Source: CAD feature listing. Evaluate the final solid. Frame: model axes, mm. Face numbers are marked on the shaded views. A direction names the side the tool comes from. Round coordinates to 2 decimals unless told otherwise and drop trailing zeros. Loops run counter-clockwise (first coordinate to the right, second up) from the corner with the lowest first, then second, coordinate; pieces in that order, holes last. Notation, with made-up numbers: (50.5, 89) -> (56.5, 89) arc R18 cw to (56.5, 98) -> close; hole circle Ø2 at (-24, -14.75). An arc over 180 degrees is marked (long way). Write item = value, one per line.
from build123d import *

# Parameters (mm, degrees)
SKETCH1_W               = 54
SKETCH1_H               = 60
BOSS_EXTRUDE1_DEPTH     = 5
BOSS_EXTRUDE2_DEPTH     = 54
SKETCH6_W               = 9.25
SKETCH6_H               = 32
CUT_EXTRUDE1_DEPTH      = 99.244592727
SKETCH8_W               = 9.25
SKETCH8_H               = 42
CUT_EXTRUDE3_DEPTH      = 99.244592727
M4_CLEARANCE_HOLE2_D    = 4.3
CUT_EXTRUDE4_DEPTH      = 94.480278669
SKETCH12_W              = 21.2
SKETCH12_H              = 46
CUT_EXTRUDE5_DEPTH      = 99.244592727
CHAMFER1_SIZE           = 2
CHAMFER2_SIZE           = 5
CHAMFER2_SIZE_2         = 5.352523158
SKETCH13_W              = 21.2
SKETCH13_H              = 5
CUT_EXTRUDE6_DEPTH      = 99.244592727
CHAMFER3_SIZE           = 5
BOSS_EXTRUDE3_DEPTH     = 19
CUT_EXTRUDE7_DEPTH      = 94.480278669
CUT_EXTRUDE7_DEPTH_BACK = 94.480278669
CHAMFER4_SIZE           = 0.4
CHAMFER5_SIZE           = 0.4


with BuildPart() as part:
    # Sketch1 → Boss-Extrude1 (new body)
    with BuildSketch(Plane.XY):
        with Locations((27, 30)):
            Rectangle(SKETCH1_W, SKETCH1_H)
    extrude(amount=BOSS_EXTRUDE1_DEPTH)

    # Sketch5 → Boss-Extrude2 (add)
    with BuildSketch(Plane.ZY):
        Polygon((56, 60), (5, 60), (5, 0), (56, 51), align=None)
    extrude(amount=-BOSS_EXTRUDE2_DEPTH)

    # Sketch6 → Cut-Extrude1 (cut, through all)
    with BuildSketch(Plane(origin=(0, 60, 0), x_dir=(1, 0, 0), z_dir=(0, 1, 0))):
        with Locations((4.625, -21)):
            Rectangle(SKETCH6_W, SKETCH6_H)
    cut_extrude1 = extrude(amount=-CUT_EXTRUDE1_DEPTH, mode=Mode.SUBTRACT)

    # Sketch8 → Cut-Extrude3 (cut, through all)
    with BuildSketch(Plane(origin=(0, 0, 0), x_dir=(-1, 0, 0), z_dir=(0, 0, -1))):
        with Locations((-4.625, 30)):
            Rectangle(SKETCH8_W, SKETCH8_H)
    cut_extrude3 = extrude(amount=-CUT_EXTRUDE3_DEPTH, mode=Mode.SUBTRACT)

    # Mirror1: Cut-Extrude1, Cut-Extrude3 across plane
    add(cut_extrude1.mirror(Plane(origin=(27, 0, 0), x_dir=(0, 0, 1), z_dir=(1, 0, 0))), mode=Mode.SUBTRACT)
    add(cut_extrude3.mirror(Plane(origin=(27, 0, 0), x_dir=(0, 0, 1), z_dir=(1, 0, 0))), mode=Mode.SUBTRACT)

    # M4 Clearance Hole2 (through all)
    with Locations(Plane(origin=(0, 0, 0), x_dir=(-1, 0, 0), z_dir=(0, 0, -1))):
        with Locations((-4.5, 55.5), (-49.5, 55.5), (-49.5, 4.5), (-4.5, 4.5)):
            Hole(M4_CLEARANCE_HOLE2_D / 2)

    # Sketch11 → Cut-Extrude4 (cut, through all)
    with BuildSketch(Plane.ZY.offset(-9.25)):
        Polygon((0, 9), (37, 51), (0, 51), align=None)
    extrude(amount=-CUT_EXTRUDE4_DEPTH, mode=Mode.SUBTRACT)

    # Sketch12 → Cut-Extrude5 (cut, through all)
    with BuildSketch(Plane(origin=(0, 60, 0), x_dir=(1, 0, 0), z_dir=(0, 1, 0))):
        with Locations((27, -28)):
            Rectangle(SKETCH12_W, SKETCH12_H)
    extrude(amount=-CUT_EXTRUDE5_DEPTH, mode=Mode.SUBTRACT)

    # Chamfer1
    chamfer1_edges = [part.edges().sort_by_distance(p)[0] for p in [
        (0, 60, 2.5),
        (0, 9, 2.5),
        (0, 51, 2.5),
        (0, 51, 46.5),
        (54, 60, 2.5),
        (0, 60, 46.5),
        (54, 60, 46.5),
        (54, 0, 2.5),
        (0, 0, 2.5),
        (54, 51, 46.5),
        (54, 9, 2.5),
        (54, 51, 2.5),
    ]]
    chamfer(chamfer1_edges, length=CHAMFER1_SIZE)

    # Chamfer2
    # the kernel refuses this chamfer: 5.352523158, 5 mm, written as the material it adds along each edge
    with BuildSketch(Plane(origin=(37.6, 51, 37), x_dir=(0, -0.7759635654606418, -0.6307777303278932), z_dir=(1, 0, 0)), Plane(origin=(9.25, 51, 37), x_dir=(0, -0.7759635654606418, -0.6307777303278932), z_dir=(1, 0, 0))) as chamfer2_piece_1:
        Polygon((CHAMFER2_SIZE * 0.999214586642, CHAMFER2_SIZE * 0.039625873385), (CHAMFER2_SIZE_2 * 0.630777730356, CHAMFER2_SIZE_2 * 0.775963565495), (0, 0), align=None)
    extrude(amount=7.15)

    # Sketch13 → Cut-Extrude6 (cut, through all)
    with BuildSketch(Plane(origin=(0, 0, 0), x_dir=(-1, 0, 0), z_dir=(0, 0, -1))):
        with Locations((-27, 48.5)):
            Rectangle(SKETCH13_W, SKETCH13_H)
    extrude(amount=-CUT_EXTRUDE6_DEPTH, mode=Mode.SUBTRACT)

    # Chamfer3
    chamfer3_edges = [part.edges().sort_by_distance(p)[0] for p in [
        (16.4, 55.5, 5),
        (16.4, 7.337837838, 5),
        (37.6, 7.337837838, 5),
        (37.6, 55.5, 5),
        (16.4, 55.5, 51),
        (37.6, 55.5, 51),
    ]]
    chamfer(chamfer3_edges, length=CHAMFER3_SIZE)

    # Sketch14 → Boss-Extrude3 (add)
    with BuildSketch(Plane(origin=(0, 0, 37), x_dir=(-1, 0, 0), z_dir=(0, 0, -1))):
        Polygon((-2, 51), (-9.25, 43.75), (-9.25, 51), align=None)
    boss_extrude3 = extrude(amount=-BOSS_EXTRUDE3_DEPTH)

    # Mirror3: Boss-Extrude3 across plane
    add(boss_extrude3.mirror(Plane(origin=(27, 0, 0), x_dir=(0, 0, 1), z_dir=(1, 0, 0))))

    # Sketch15 → Cut-Extrude7 (cut, two sides: drawn at the far end of the back side and taken through both)
    with BuildSketch(Plane(origin=(9.25, 0, 0), x_dir=(0, 0, -1), z_dir=(1, 0, 0)).offset(-CUT_EXTRUDE7_DEPTH_BACK)):
        Polygon((-48.75, 43.75), (-56, 51), (-56, 43.75), align=None)
    extrude(amount=CUT_EXTRUDE7_DEPTH + CUT_EXTRUDE7_DEPTH_BACK, mode=Mode.SUBTRACT)

    # Chamfer4
    chamfer4_edges = [part.edges().sort_by_distance(p)[0] for p in [
        (47.35, 55.5, 37),
        (47.35, 55.5, 56),
        (2.35, 55.5, 56),
        (2.35, 55.5, 37),
    ]]
    chamfer(chamfer4_edges, length=CHAMFER4_SIZE)

    # Chamfer5
    chamfer5_edges = [part.edges().sort_by_distance(p)[0] for p in [
        (2.35, 4.5, 5),
        (2.35, 4.5, 0),
        (47.35, 4.5, 5),
        (47.35, 4.5, 0),
        (47.35, 55.5, 5),
        (47.35, 55.5, 0),
        (2.35, 55.5, 5),
        (2.35, 55.5, 0),
    ]]
    chamfer(chamfer5_edges, length=CHAMFER5_SIZE)


solid = part.part
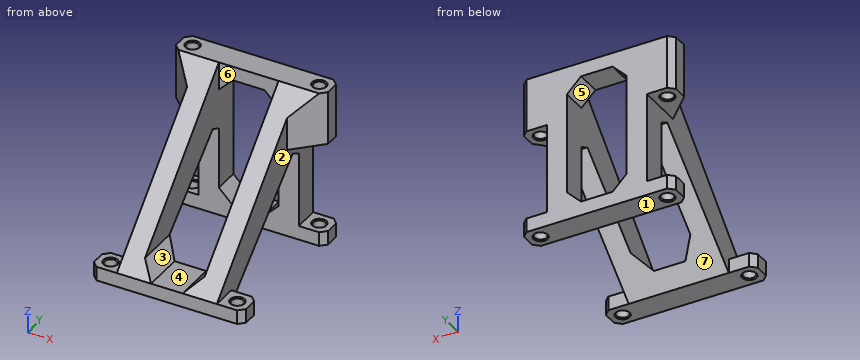
1. Section query A-A (z = 45). Return the cut outline in (x, y).
Evaluation:
outline = (0, 53) -> (9.25, 43.75) -> (9.25, 40) -> (16.4, 40) -> (16.4, 60) -> (2, 60) -> (0, 58) -> close; (37.6, 40) -> (44.75, 40) -> (44.75, 43.75) -> (54, 53) -> (54, 58) -> (52, 60) -> (37.6, 60) -> close; hole circle Ø4.3 at (4.5, 55.5); hole circle Ø4.3 at (49.5, 55.5)
2. Section query D-D (y = 55.5). Give the number of separate pieces and of enclosed holes in the cut face, then the cut area to 3 significant figures.
Evaluation:
separate_pieces = 5
enclosed_holes = 1
area = 1,300 mm²
3. Set-up query: the marked faces 4, 5, 6 and 7. Return all of +Z, -Z, +X, -X, +Y, -Y with unobstructed straight access to the full face (end or side cutting, diameter ignored); none if empty.
Evaluation:
face_4 = +Z, +Y, -Y
face_5 = +Y, -Y
face_6 = +Z, -Z, -Y
face_7 = -Z, +X, -X
4. Mould query, pull axis Z, two halves, no side actions, for the marked faces 1, 2 and 3. Classes: released by +Z, released by -Z, zero draft, split by the parting line, or undercut.
Evaluation:
face_1 = released by -Z
face_2 = undercut
face_3 = released by +Z
5. Section query C-C (z = 36). Return the cut outline in (x, y).
Evaluation:
outline = (9.25, 31) -> (16.4, 31) -> (16.4, 60) -> (9.25, 60) -> close; (37.6, 31) -> (44.75, 31) -> (44.75, 60) -> (37.6, 60) -> close
6. Line query: probe 1 along Y at (x, z) = (49.5, 2.15); probe 2 along Z at (x, y) = (30, 52.5); probe 3 along X at (y, z) = (55, 50). Output: solid intervals per line, ascending. Write a range as from..to.
Evaluation:
probe_1 = 0..2.35, 6.65..9, 51..53.35, 57.65..60
probe_2 = 0..5, 51..56
probe_3 = 0..2.41, 6.59..20.4, 33.6..47.41, 51.59..54
7. Contact query for flat-ended pins moving along their axis: pin 1 Ø14 at (y, z) = (40, 36) entering from -X; pin 2 Ø5 at (x, y) = (49.5, 55.5) entering from +Z; pin 3 Ø1.5 at (x, z) = (15.5, 39.5) entering from -Y. Output: stop coordinate, or through.
Evaluation:
pin_1 = 6.07
pin_2 = 55.95
pin_3 = 33.75
8. Section query B-B (x = 23). Return the cut outline in (y, z), then the cut area to 3 significant figures.
Evaluation:
outline = (0, 0) -> (9, 0) -> (14.68, 5) -> (0, 5) -> close; (51, 0) -> (60, 0) -> (60, 5) -> (51, 5) -> close; (51, 51) -> (60, 51) -> (60, 56) -> (51, 56) -> close
area = 149 mm²
